from build123d import *

# Parameters (mm, degrees)
F0_R     = 3
F0_R_2   = 12.5
F0_R_3   = 7.5
F1_DEPTH = 30


with BuildPart() as f1:
    # F0 (on Front) → F1 (new body)
    with BuildSketch(Plane.XZ):
        Polygon((4.39074, 26.841277), (-45.60926, 26.841277), (-45.60926, -23.158723), (54.39074, -23.158723), (54.39074, 1.841277), (4.39074, 1.841277), align=None)
        with Locations((-39.60926, -17.158723)):
            Circle(F0_R, mode=Mode.SUBTRACT)
        with Locations((-1.60926, -17.158723)):
            Circle(F0_R, mode=Mode.SUBTRACT)
        with Locations((-20.60926, 1.841277)):
            Circle(F0_R_2, mode=Mode.SUBTRACT)
        with Locations((34.39074, -10.658723)):
            Circle(F0_R_3, mode=Mode.SUBTRACT)
        with Locations((-39.60926, 20.841277)):
            Circle(F0_R, mode=Mode.SUBTRACT)
        with Locations((-1.60926, 20.841277)):
            Circle(F0_R, mode=Mode.SUBTRACT)
    extrude(amount=F1_DEPTH)


solid = f1.part
Model file for the job. Use its own axes, mm. A direction names the side the tool comes from. Coordinates: 2 decimals unless noted, no trailing zeros. Order: outer loops, then holes, each group sorted by start corner. A loop starts at its lowest first (then second) coordinate and runs counter-clockwise, first axis right, second up. Notation, with made-up numbers: (55.5, 48.25) -> (92.5, 48.25) arc R25 ccw to (92.5, 84.25) -> close; hole circle Ø9 at (8.5, 11.5). An arc over 180 degrees is marked (long way). Return JSON: item names as keys, results as strings. Group by question number.
Item 1: Saw through at D-D on y = -8. Write the cut outline in (x, z).
Item 2: Tool access for faces 1 (the flat face through (54.391, -15, -11)), 2 (the flat face through (30, -15, 1.841)): list every direction of +Z, -Z, +X, -X, +Y, -Y with a clear straight run to the whole face (end or side of a thin tool).
Item 3: Saw through at C-C on z = 10.5. Write the cut outline in (x, y), then the cut area to 3 significant figures.
Item 4: Flat gauge pins, fed straight in: P1, Ø9, axis at x = 34.39, z = -10.66, coming from the -Y side; P2, Ø6, axis at y = -7, z = 9.5, coming from the +X side; P3, Ø6, axis at x = 29, z = -12, coming from the +Y side. Where does each tip first touch, or does it go through?
Item 5: Pull direction X, two halves, no side cores. Call faces 3 (the flat face through (4.391, -15, 14)), 4 (the cylindrical face through (-2.26, -14.79, -20.087)), 5 (the flat face through (-7, -30, -3)): pulls with the +X half, pulls with the -X half, needs draft (parallel to the pull), parting line crosses it, or undercut.
Item 6: Wall check: line 1 along Z through (x, y) = (-1.5, -3.75); line 2 along X through (y, z) = (-8, 23.5); line 3 along Z through (x, y) = (-2.5, -7.5). Give the ranges that are in metal, low to high. Write a range as [from, to].
Item 7: Saw through at A-A on z = -8.5. Write the cut outline in (x, y), then the cut area to 3 significant figures.
Item 8: Saw through at B-B on x = 29. Write the cut outline in (y, z), then the cut area to 3 significant figures.
Values found:
{
 "1": {"outline": "(-45.61, -23.16) -> (54.39, -23.16) -> (54.39, 1.84) -> (4.39, 1.84) -> (4.39, 26.84) -> (-45.61, 26.84) -> close; hole circle Ø6 at (-39.61, -17.16); hole circle Ø6 at (-39.61, 20.84); hole circle Ø25 at (-20.61, 1.84); hole circle Ø6 at (-1.61, -17.16); hole circle Ø6 at (-1.61, 20.84); hole circle Ø15 at (34.39, -10.66)"},
 "2": {"face 1": "+Z, -Z, +X, +Y, -Y", "face 2": "+Z, +X, +Y, -Y"},
 "3": {"outline": "(-45.61, -30) -> (-29.62, -30) -> (-29.62, 0) -> (-45.61, 0) -> close; (-11.59, -30) -> (4.39, -30) -> (4.39, 0) -> (-11.59, 0) -> close", "area": "959 mm2"},
 "4": {"P1": "passes through", "P2": "stops at x = 4.39", "P3": "stops at y = 0"},
 "5": {"face 3": "pulls with the +X half", "face 4": "undercut", "face 5": "needs draft"},
 "6": {"line 1": "z = [-23.16, -20.16], [-14.16, 17.84], [23.84, 26.84]", "line 2": "x = [-45.61, -41], [-38.22, -3], [-0.22, 4.39]", "line 3": "z = [-23.16, -20.02], [-14.29, 17.98], [23.71, 26.84]"},
 "7": {"outline": "(-45.61, -30) -> (-27.63, -30) -> (-27.63, 0) -> (-45.61, 0) -> close; (-13.59, -30) -> (27.21, -30) -> (27.21, 0) -> (-13.59, 0) -> close; (41.57, -30) -> (54.39, -30) -> (54.39, 0) -> (41.57, 0) -> close", "area": "2,150 mm2"},
 "8": {"outline": "(-30, -23.16) -> (0, -23.16) -> (0, -15.87) -> (-30, -15.87) -> close; (-30, -5.44) -> (0, -5.44) -> (0, 1.84) -> (-30, 1.84) -> close", "area": "437 mm2"}
}
